Check sheet for the modelled part. Datum: model origin and axes. Units: mm. Face numbers are marked on the shaded views. A direction names the side the tool comes from. Give positions to 0.01 mm unless a question says otherwise; leave off trailing zeros. Loops run counter-clockwise (first coordinate to the right, second up) from the corner with the lowest first, then second, coordinate; pieces in that order, holes last. Notation, with made-up numbers: (4, 34) - (61, 34) arc R14 cw to (61, 38) - close; hole circle Ø9 at (45, -29.5). An arc over 180 degrees is marked (long way). Use one line per item in the form item = value.
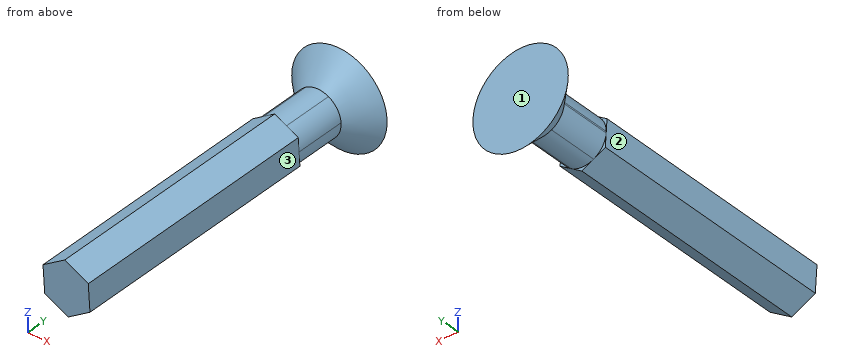
from build123d import *

# Parameters (mm, degrees)
F1_DEPTH  = 150
F3_DEPTH  = 30
F3_FACE_R = 13.5946213818
F4_DEPTH  = 15
F4_TAPER  = -45


with BuildPart() as f1:
    # F0 (on Front) → F1 (new body)
    with BuildSketch(Plane.XZ):
        Polygon((13.0521743593, 8.7211840853), (-1.0266797893, 15.6641066124), (-14.0788541486, 6.9429225271), (-13.0521743593, -8.7211840853), (1.0266797893, -15.6641066124), (14.0788541486, -6.9429225271), align=None)
    extrude(amount=F1_DEPTH)

    # F2 (on face) → F3 (join)
    with BuildSketch(Plane(origin=(0, 0, 0), x_dir=(-1, 0, 0), z_dir=(0, 1, 0))):
        with BuildLine():
            ThreePointArc((13.5655142354, -0.8891310612), (13.5873426467, -0.4448036842), (13.5946213818, 0))
            ThreePointArc((13.5946213818, 0), (11.9893857748, 6.4084599756), (7.5527673124, 11.3035143403))
            ThreePointArc((7.5527673124, 11.3035143403), (0.8891311409, 13.5655142302), (-6.012747005, 12.1926454869))
            ThreePointArc((-6.012747005, 12.1926454869), (-11.3035143729, 7.5527672636), (-13.565514228, 0.8891311747))
            ThreePointArc((-13.565514228, 0.8891311747), (-12.1926455438, -6.0127468897), (-7.5527673722, -11.3035143003))
            ThreePointArc((-7.5527673722, -11.3035143003), (-0.8891308824, -13.5655142471), (6.0127475341, -12.192645226))
            ThreePointArc((6.0127475341, -12.192645226), (11.3035145684, -7.552766971), (13.5655142354, -0.8891310612))
        make_face()
    extrude(amount=F3_DEPTH)

    # F3_face (on face) → F4 (join)
    with BuildSketch(Plane(origin=(0, 30, 0), x_dir=(-1, 0, 0), z_dir=(0, 1, 0))):
        Circle(F3_FACE_R)
    extrude(amount=F4_DEPTH, taper=F4_TAPER)


solid = f1.part
Item 1: Thickness scan on L1, parallel to X at y = -109.5, z = 0; L2, parallel to Z at x = -8.5, y = -125; L3, parallel to X at y = -100.5, z = -3. Record the ranges inside material, lowest first.
Answer block:
L1 = -13.62 to 13.62
L2 = -10.97 to 10.67
L3 = -13.43 to 13.82
Item 2: Gauge pin test, flat ends, axial feed: P1, Ø1, axis at y = -14.5, z = -15, coming from the -X side; P2, Ø2, axis at x = -22, z = 4.5, coming from the -Y side; P3, Ø3, axis at x = 6.5, y = -42, coming from the -Z side. Record the tip position at first contact, or that the pin passes through.
Answer block:
P1 = -1.33
P2 = 37.86
P3 = -13.01
Item 3: Access from +Z, -Z, +X, -X, +Y, -Y to the whole of each face (thin tool, end or side, straight path). Record for the marked faces 1, 2 and 3.
Answer block:
face_1 = +Z, -Z, +X, -X, +Y
face_2 = -Z, -X, -Y
face_3 = +Z, +X, -Y
Item 4: Section check A-A on y = -91. Record the boundary of the cut face in (x, z), then the cut area to 3 significant figures.
Answer block:
outline = (-14.08, 6.94) - (-13.05, -8.72) - (1.03, -15.66) - (14.08, -6.94) - (13.05, 8.72) - (-1.03, 15.66) - close
area = 640 mm2
